Autodesk Inventor part; units mm, degrees
ref_plane "YZ Plane" through (0, 0, 0) normal (1, 0, 0) x (0, 1, 0)
ref_plane "XZ Plane" through (0, 0, 0) normal (0, 1, 0) x (-1, 0, 0)
ref_plane "XY Plane" through (0, 0, 0) normal (0, 0, 1) x (1, 0, 0)
sketch "草圖1" plane through (0, 0, 0) normal (0, 0, 1) x (1, 0, 0)
  line L0 (-50, -10) -> (50, -10)
  line L1 (50, -10) -> (50, 10)
  line L2 (50, 10) -> (-50, 10)
  line L3 (-50, 10) -> (-50, -10)
  line L4 (-50, -10) -> (50, 10) construction
  line L5 (50, -10) -> (-50, 10) construction
  point P0 (0, 0)
  dimension "d0" = 20
  dimension "d1" = 100
extrude "擠出1" add sketch "草圖1" along normal blind 15
sketch "草圖2" plane through (50, -10, 0) normal (1, 0, 0) x (0, 0, -1)
  circle A0 centre (-15, 10) radius 8
  line L0 (0, 0) -> (0, 20)
  point P0 (0, 10)
  dimension "d4" = 16
  dimension "d5" = 15
sketch "草圖3" plane through (-50, -10, 0) normal (-1, 0, 0) x (0, 0, 1)
  circle A0 centre (12, 10) radius 9
  line L0 (0, 20) -> (0, 0)
  point P0 (0, 10)
  dimension "d6" = 18
  dimension "d7" = 12
sketch "草圖4" plane through (0, 0, 15) normal (0, 0, 1) x (1, 0, 0)
  line L0 (49.8919, 0) -> (-50, 0)
  line L1 (-50, 10) -> (-50, -10)
  point P0 (0, 0)
loft "斷面混成1" cut profiles "草圖3", "草圖2"
sketch "草圖5" plane through (0, 0, 0) normal (0, 0, -1) x (-1, 0, 0)
  circle A0 centre (25, 0) radius 5
  circle A1 centre (-25, 0) radius 5
  point P0 (0, 0)
  dimension "d12" = 10
  dimension "d13" = 10
  dimension "d14" = 50
  dimension "d15" = 25
extrude "擠出2" add sketch "草圖5" along normal blind 20
properties part number "滑軌2"
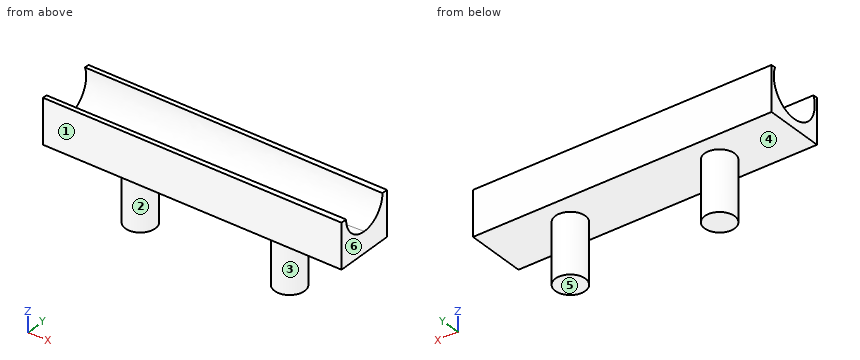
Can you work these out from the model? Positions are in its coordinate system, mm. Face numbers are marked on the shaded views. A direction names the side the tool comes from. Give positions to 0.01 mm unless a question says otherwise; leave off trailing zeros. Loops run counter-clockwise (first coordinate to the right, second up) from the corner with the lowest first, then second, coordinate; pieces in that order, holes last. Notation, with made-up numbers: (-31.5, 83) -> (21.5, 83) arc R19 ccw to (21.5, 105) -> close; hole circle Ø5 at (77, 60.25). An arc over 180 degrees is marked (long way). Use one line per item in the form item = value.
1) If we section it at A-A (z = -3.5): Please give me the cut outline in (x, y), plus the area to 3 significant figures.
Answers:
outline = circle Ø10 at (-25, 0); circle Ø10 at (25, 0)
area = 157 mm²
2) I need wall thicknesses on line 1 along Y through (x, z) = (-1, 11); line 2 along Y through (x, z) = (-9, 6); line 3 along X through (y, z) = (4, -1). Which ranges of each line are inside material? Lowest first, please.
Answers:
line_1 = -10 to -8.14, 8.14 to 10
line_2 = -10 to -4.64, 4.64 to 10
line_3 = -28 to -22, 22 to 28
3) For the marked faces 1 and 2, which set-ups out of +Z, -Z, +X, -X, +Y, -Y let a thin tool reach every point of the face, with its end or its side?
Answers:
face_1 = +Z, -Z, +X, -X, -Y
face_2 = -Z
4) Will these pins go through, and if not, where does the flat tip stop? pin 1 (3 mm diameter, centred on x = 25, z = -15.5, fed in from -Y); pin 2 (3 mm diameter, centred on x = -2, y = 6, fed in from +Z); pin 3 (10 mm diameter, centred on y = -0.5, z = -9, fed in from +X).
Answers:
pin_1 = -5
pin_2 = 9.4
pin_3 = 30
5) We'd pull the mould along X, two halves only. Please class the marked faces 3, 4, 5 and 6: released by +X, released by -X, zero draft, split by the parting line, or undercut.
Answers:
face_3 = undercut
face_4 = undercut
face_5 = zero draft
face_6 = released by +X
